```python
from build123d import *

# Parameters (mm, degrees)
CROQUIS1_R              = 1.6
SALIENTE_EXTRUIR1_DEPTH = 3


with BuildPart() as part:
    # Croquis1 → Saliente-Extruir1 (new body)
    with BuildSketch(Plane(origin=(0, 0, 0), x_dir=(1, 0, 0), z_dir=(0, 1, 0))):
        with BuildLine():
            Line((-0.5, 0), (-5, 0))
            Line((-5, 0), (-5, -5))
            Line((-5, -5), (5, -5))
            Line((5, -5), (5, 5))
            Line((5, 5), (0, 5))
            Line((0, 5), (0, 0.5))
            ThreePointArc((0, 0.5), (0.353553391, -0.353553391), (-0.5, 0))
        make_face()
        with Locations(Location((-2.5, -2.5, 0), (0, 0, 270))):
            Circle(CROQUIS1_R, mode=Mode.SUBTRACT)
        with Locations(Location((2.5, 2.5, 0), (0, 0, 270))):
            Circle(CROQUIS1_R, mode=Mode.SUBTRACT)
    extrude(amount=SALIENTE_EXTRUIR1_DEPTH)


solid = part.part
```
Part model, mm, in its own coordinate system. A direction names the side the tool comes from. Give positions to 0.01 mm unless a question says otherwise; leave off trailing zeros. Order: outer loops, then holes, each group sorted by start corner. A loop starts at its lowest first (then second) coordinate and runs counter-clockwise, first axis right, second up. Notation, with made-up numbers: M 67,67.5 L 75,67.5 A19 ccw 75,94.5 Z; hole C 38.25,27 d2. An arc over 180 degrees is marked long. Use a Markdown table: item, result. Add a question column.
(1) Saw through at C-C, the plane y = 2.65. Give the cut face in (x, z).
(2) Saw through at B-B, the plane z = -2.5. Give the cut face in (x, y).
(3) Drop flat-ended pins along their axis: P1, Ø3.5, axis at x = 2.5, z = -2.5, coming from the +Y side; P2, Ø1.5, axis at x = -3, y = 2, coming from the -Z side. Give the stop position or say it passes through.
(4) Probe line 1 along X through (y, z) = (1.5, 2.5); line 2 along X through (y, z) = (1.35, 1.75); line 3 along Z through (x, y) = (-3.25, 1.1). List the from-to ranges inside material, lowest first. Write a range as [from, to].
(5) Mould opens along Z. For faces 1 (the face through (1, 0, 1)), 2 (the face through (0.4, 1.5, 0.3)), 3 (the face through (0, 1, 5)), 4 (the face through (-4.06, 1.48, 2.15)) say: +Z half, -Z half, draft (parallel to the pull), parting line (faces both ways), or undercut.
(6) 3-axis set-ups, long thin cutter, end or side, ignore diameter. For faces 5 (the face through (-3, 1, 0)), 6 (the face through (3, 1, -5)): which of +Z, -Z, +X, -X, +Y, -Y reach the whole face in a straight line?
(7) Saw through at A-A, the plane x = -2.5. Give the cut face in (y, z).
Answer key:
| question | item | result |
|---|---|---|
| 1 | outline | M -5,0 L -0.5,0 A0.5 cw long 0,-0.5 L 0,-5 L 5,-5 L 5,5 L -5,5 Z; hole C -2.5,2.5 d3.2; hole C 2.5,-2.5 d3.2 |
| 2 | outline | M 0,0 L 0.9,0 L 0.9,3 L 0,3 Z; M 4.1,0 L 5,0 L 5,3 L 4.1,3 Z |
| 3 | P1 | y = 3 |
| 3 | P2 | z = 0 |
| 4 | line 1 | [-5, -4.1], [-0.9, 5] |
| 4 | line 2 | [-5, -3.91], [-1.09, 5] |
| 4 | line 3 | [0, 1.09], [3.91, 5] |
| 5 | face 1 | draft |
| 5 | face 2 | undercut |
| 5 | face 3 | +Z half |
| 5 | face 4 | undercut |
| 6 | face 5 | -Z, -X, +Y, -Y |
| 6 | face 6 | -Z, +X, -X, +Y, -Y |
| 7 | outline | M 0,0 L 3,0 L 3,0.9 L 0,0.9 Z; M 0,4.1 L 3,4.1 L 3,5 L 0,5 Z |
